Geometry check sheet. Reference: the model listing, model coordinates, mm. A direction names the side the tool comes from. Give positions to 0.01 mm unless a question says otherwise; leave off trailing zeros. Order: outer loops, then holes, each group sorted by start corner. A loop starts at its lowest first (then second) coordinate and runs counter-clockwise, first axis right, second up. Notation, with made-up numbers: M 32.25,44 L 82.25,44 A32 ccw 82.25,74 Z; hole C 88,-21 d9. An arc over 180 degrees is marked long. Answer as CSV lines item,"result". Start each with the question number.
Q1. Section check C-C, the plane y = 14.75. Record the boundary of the cut face in (x, z).
Q2. Set-up check for faces 4 (the flat face through (-28.75, 0, -4)), 5 (the flat face through (-60.397, 13, 5)), 6 (the flat face through (-38.75, 0, -4)), 7 (the flat face through (-30, 27.301, 6)): record each of +Z, -Z, +X, -X, +Y, -Y from which the full face is reachable in a straight line by a thin tool's end or side.
Q3. Section check A-A, the plane x = -22. Record the boundary of the cut face in (y, z).
Q4. Thickness scan on line 1 (X direction, y = 0.25, z = 1.25); line 2 (Y direction, x = -50, z = 9); line 3 (Z direction, x = -42.5, y = 22.25). Record the ranges inside material, lowest first.
Q5. Section check B-B, the plane z = 9. Record the boundary of the cut face in (x, y).
Q6. Section check D-D, the plane x = -32. Record the boundary of the cut face in (y, z).
Q7. Go/stop test with flat-tipped pins: pin 1 (2 mm diameter, centred on y = 0, z = -4.5, fed in from -X); pin 2 (1 mm diameter, centred on x = -56.5, y = 27, fed in from -Z); pin 3 (2 mm diameter, centred on x = -11.5, y = 11.5, fed in from -Z). Record where each tip stops, or that it passes through.
Q8. Mould release check, pull along X, two halves, no side actions. Record for faces 1 (the flat face through (-31, 14, 13)), 2 (the flat face through (-30, 14, 11)), 3 (the flat face through (-28.75, 27, -4)): +X half, -X half, draft (parallel to the pull), parting line (faces both ways), or undercut.
```python
from build123d import *

# Parameters (mm, degrees)
SKETCH1_W            = 62.6472
SKETCH1_H            = 29.551
SKETCH1_W_2          = 60.6472
SKETCH1_H_2          = 27.551
BOSS_EXTRUDE1_DEPTH  = 11
CUT_EXTRUDE1_REACH   = 64.647
SKETCH4_W            = 2
SKETCH4_H            = 1
BOSS_EXTRUDE2_DEPTH  = 1
SKETCH6_W            = 2
SKETCH6_H            = 1
BOSS_EXTRUDE3_DEPTH  = 1
BOSS_EXTRUDE4_START  = -30
SKETCH7_W            = 1
SKETCH7_H            = 1
BOSS_EXTRUDE4_DEPTH  = 10
BOSS_EXTRUDE5_START  = 40
SKETCH9_W            = 1
SKETCH9_H            = 1.5
BOSS_EXTRUDE5_DEPTH  = 10
BOSS_EXTRUDE7_START  = -30
BOSS_EXTRUDE7_DEPTH  = 10
SKETCH12_W           = 62.6472
SKETCH12_H           = 29.551
BOSS_EXTRUDE8_DEPTH  = 2
BOSS_EXTRUDE9_DEPTH  = 1
BOSS_EXTRUDE10_START = -29.551
BOSS_EXTRUDE10_DEPTH = 1


with BuildPart() as part:
    # Sketch1 → Boss-Extrude1 (new body)
    with BuildSketch(Plane.XY):
        with Locations((-30.0736, 13.5255)):
            Rectangle(SKETCH1_W, SKETCH1_H)
        with Locations((-30.0736, 13.5255)):
            Rectangle(SKETCH1_W_2, SKETCH1_H_2, mode=Mode.SUBTRACT)
    extrude(amount=BOSS_EXTRUDE1_DEPTH)

    # Sketch3 → Cut-Extrude1 (cut, up to next)
    with BuildSketch(Plane.ZY.offset(61.3972), mode=Mode.PRIVATE) as cut_extrude1_sk1:
        Polygon((0, 17.5514), (0.75, 18.3233), (0.75, 24.3233), (0, 25.0952), align=None)
    cut_extrude1_tool1 = extrude(cut_extrude1_sk1.sketch, amount=-CUT_EXTRUDE1_REACH, mode=Mode.PRIVATE) & part.part
    add(cut_extrude1_tool1.solids().sort_by_distance((-61.3972, 21.3233, 0.360752))[0], mode=Mode.SUBTRACT)

    # Sketch4 → Boss-Extrude2 (add)
    with BuildSketch(Plane(origin=(0, -0.25, 0), x_dir=(1, 0, 0), z_dir=(0, 1, 0))):
        with Locations((-54.3972, -2.3375)):
            Rectangle(SKETCH4_W, SKETCH4_H)
        with Locations((-5.75, -2.3375)):
            Rectangle(SKETCH4_W, SKETCH4_H)
    extrude(amount=BOSS_EXTRUDE2_DEPTH)

    # Sketch6 → Boss-Extrude3 (add)
    with BuildSketch(Plane.XZ.offset(-27.301)):
        with Locations((-2.75, 2.3375)):
            Rectangle(SKETCH6_W, SKETCH6_H)
        with Locations((-51.3776, 2.783222425)):
            Rectangle(SKETCH6_W, SKETCH6_H)
    extrude(amount=BOSS_EXTRUDE3_DEPTH)

    # Sketch7 → Boss-Extrude4 (add)
    with BuildSketch(Plane(origin=(1.25, 0, 0), x_dir=(0, 0, -1), z_dir=(1, 0, 0)).offset(BOSS_EXTRUDE4_START)):
        with Locations((0.5, 27.451)):
            Rectangle(SKETCH7_W, SKETCH7_H)
    extrude(amount=-BOSS_EXTRUDE4_DEPTH)

    # Sketch9 → Boss-Extrude5 (add)
    with BuildSketch(Plane.ZY.offset(-1.25).offset(BOSS_EXTRUDE5_START)):
        with Locations((-0.5, -0.5)):
            Rectangle(SKETCH9_W, SKETCH9_H)
    extrude(amount=-BOSS_EXTRUDE5_DEPTH)

    # Sketch11 → Boss-Extrude7 (add)
    with BuildSketch(Plane(origin=(1.25, 0, 0), x_dir=(0, 0, -1), z_dir=(1, 0, 0)).offset(BOSS_EXTRUDE7_START)):
        Polygon((5, 28.301), (5, 27.301), (3.25, 25.551), (3.25, 27.301), (0, 27.301), (0, 28.301), align=None)
        Polygon((0, -1.25), (5, -1.25), (5, -0.25), (3.25, 1.5), (3.25, -0.25), (0, -0.25), align=None)
    extrude(amount=-BOSS_EXTRUDE7_DEPTH)

    # Sketch12 → Boss-Extrude8 (add)
    with BuildSketch(Plane.XY.offset(11)):
        with Locations((-30.0736, 13.5255)):
            Rectangle(SKETCH12_W, SKETCH12_H)
    extrude(amount=BOSS_EXTRUDE8_DEPTH)

    # Sketch13 → Boss-Extrude9 (add)
    with BuildSketch(Plane.XZ.offset(1.25)):
        with BuildLine():
            Line((-25.75, 0), (-28.75, 0))
            Line((-28.75, 0), (-28.75, -3))
            ThreePointArc((-28.75, -3), (-27.871320344, -0.878679656), (-25.75, 0))
        make_face()
        with BuildLine():
            Line((-41.75, 0), (-38.75, 0))
            Line((-38.75, 0), (-38.75, -3))
            ThreePointArc((-38.75, -3), (-39.628679656, -0.878679656), (-41.75, 0))
        make_face()
    extrude(amount=-BOSS_EXTRUDE9_DEPTH)

    # Sketch13<2> → Boss-Extrude10 (add)
    with BuildSketch(Plane.XZ.offset(1.25).offset(BOSS_EXTRUDE10_START)):
        with BuildLine():
            Line((-25.75, 0), (-28.75, 0))
            Line((-28.75, 0), (-28.75, -3))
            ThreePointArc((-28.75, -3), (-27.871320344, -0.878679656), (-25.75, 0))
        make_face()
        with BuildLine():
            Line((-41.75, 0), (-38.75, 0))
            Line((-38.75, 0), (-38.75, -3))
            ThreePointArc((-38.75, -3), (-39.628679656, -0.878679656), (-41.75, 0))
        make_face()
    extrude(amount=BOSS_EXTRUDE10_DEPTH)


solid = part.part
```
Answer block:
1,outline,"M -61.4,0 L -60.4,0 L -60.4,11 L 0.25,11 L 0.25,0 L 1.25,0 L 1.25,13 L -61.4,13 Z"
2,face 4,"-Z, +X, +Y, -Y"
2,face 5,"-Z"
2,face 6,"-Z, -X, +Y, -Y"
2,face 7,"none"
3,outline,"M -1.25,0 L -0.25,0 L -0.25,11 L 27.3,11 L 27.3,0 L 28.3,0 L 28.3,13 L -1.25,13 Z"
4,line 1,"x = -61.4 to -60.4, 0.25 to 1.25"
4,line 2,"y = -1.25 to -0.25, 27.3 to 28.3"
4,line 3,"z = 11 to 13"
5,outline,"M -61.4,-1.25 L 1.25,-1.25 L 1.25,28.3 L -61.4,28.3 Z; hole M -60.4,-0.25 L 0.25,-0.25 L 0.25,27.3 L -60.4,27.3 Z"
6,outline,"M -1.25,-5 L -0.25,-5 L 1.5,-3.25 L -0.25,-3.25 L -0.25,-1 L 0.25,-1 L 0.25,0 L -0.25,0 L -0.25,11 L 27.3,11 L 27.3,0 L 26.95,0 L 26.95,-1 L 27.3,-1 L 27.3,-3.25 L 25.55,-3.25 L 27.3,-5 L 28.3,-5 L 28.3,13 L -1.25,13 Z"
7,pin 1,"stops at x = -38.75"
7,pin 2,"stops at z = 0"
7,pin 3,"stops at z = 11"
8,face 1,"draft"
8,face 2,"undercut"
8,face 3,"+X half"
